from build123d import *

# Parameters (mm, degrees)
SKETCH1_W           = 85.5
SKETCH1_H           = 85.5
BOSS_EXTRUDE1_DEPTH = 3
FILLET1_R           = 2
SKETCH3_R           = 1.85
CUT_EXTRUDE1_DEPTH  = 10
SKETCH4_R           = 2.5
SKETCH4_R_2         = 1.85
CUT_EXTRUDE2_DEPTH  = 10


with BuildPart() as part:
    # Sketch1 → Boss-Extrude1 (new body)
    with BuildSketch(Plane(origin=(0, 0, 0), x_dir=(1, 0, 0), z_dir=(0, 1, 0))):
        Rectangle(SKETCH1_W, SKETCH1_H)
    extrude(amount=BOSS_EXTRUDE1_DEPTH)

    # Fillet1
    fillet1_edges = [part.edges().sort_by_distance(p)[0] for p in [
        (-42.75, 1.5, -42.75),
        (42.75, 1.5, -42.75),
        (42.75, 1.5, 42.75),
        (-42.75, 1.5, 42.75),
    ]]
    fillet(fillet1_edges, radius=FILLET1_R)

    # Sketch3 → Cut-Extrude1 (cut)
    with BuildSketch(Plane(origin=(0, 3, 0), x_dir=(1, 0, 0), z_dir=(0, 1, 0))):
        with Locations(Location((-25, 39, 0), (0, 0, 270))):
            Circle(SKETCH3_R)
        with Locations(Location((25, 39, 0), (0, 0, 270))):
            Circle(SKETCH3_R)
        with Locations(Location((25, -39, 0), (0, 0, 270))):
            Circle(SKETCH3_R)
        with Locations(Location((-25, -39, 0), (0, 0, 270))):
            Circle(SKETCH3_R)
    extrude(amount=-CUT_EXTRUDE1_DEPTH, mode=Mode.SUBTRACT)

    # Sketch4 → Cut-Extrude2 (cut)
    with BuildSketch(Plane(origin=(0, 3, 0), x_dir=(1, 0, 0), z_dir=(0, 1, 0))):
        with Locations(Location((-12.5, 10, 0), (0, 0, 270))):
            Circle(SKETCH4_R)
        with Locations(Location((-12.5, -10, 0), (0, 0, 270))):
            Circle(SKETCH4_R)
        with Locations(Location((12.5, 10, 0), (0, 0, 270))):
            Circle(SKETCH4_R)
        with Locations(Location((12.5, -10, 0), (0, 0, 270))):
            Circle(SKETCH4_R)
        with Locations(Location((-34.25, 16.7, 0), (0, 0, 270))):
            Circle(SKETCH4_R_2)
        with Locations(Location((-34.25, -10.7, 0), (0, 0, 270))):
            Circle(SKETCH4_R_2)
        with Locations(Location((34.25, -10.7, 0), (0, 0, 270))):
            Circle(SKETCH4_R_2)
        with Locations(Location((34.25, 16.7, 0), (0, 0, 270))):
            Circle(SKETCH4_R_2)
    extrude(amount=-CUT_EXTRUDE2_DEPTH, mode=Mode.SUBTRACT)


solid = part.part
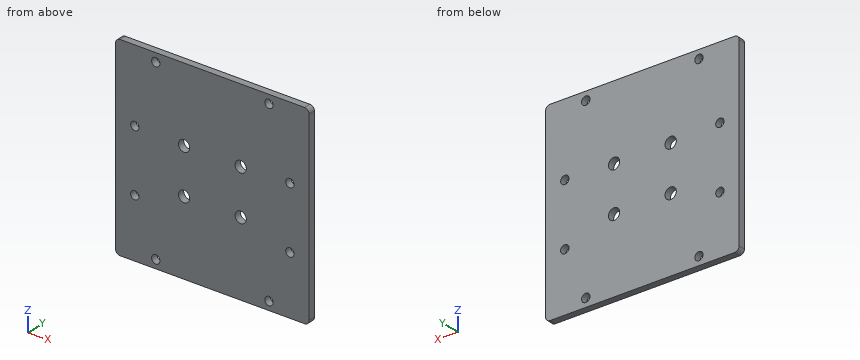
The model under review builds one solid part; all positions refer to its coordinate system, in mm. Coordinates: 2 decimals unless noted, no trailing zeros. Loops run counter-clockwise (first coordinate to the right, second up) from the corner with the lowest first, then second, coordinate; pieces in that order, holes last. Notation, with made-up numbers: M 65.25,-39 L 82.25,-39 A13 ccw 82.25,-33 Z; hole C 31.5,-39.75 d8. An arc over 180 degrees is marked long. Put each result on its own line as item: value. Start each with the question number.
Q1. Clearance check with a flat-ended pin moving along its axis: pin 1 (2 mm diameter, centred on x = 25, z = 39, fed in from +Y). State where the tip first meets the part, or that it passes through.
Q2. Add section D-D (z = 10.7). Write out the cut boundary in (x, y).
Q3. Add section B-B (z = -8.5). Write out the cut boundary in (x, y), and give its area (4 significant figures).
Q4. Add section C-C (y = 0.55). Count the separate pieces of the cut face and the enclosed holes in it, and give its area (3 significant figures).
Q5. Add section A-A (x = 12.5). Write out the cut boundary in (y, z), and give its area (4 significant figures).
Q6. Wall thickness on line 1 (Z direction, x = -13, y = 2.7); line 2 (X direction, y = 2.3, z = 10); line 3 (X direction, y = 1, z = 10.7): over which ranges is each line inside the solid? List them lowest first.
Answers:
1. pin 1: passes through
2. outline: M -42.75,0 L -36.1,0 L -36.1,3 L -42.75,3 Z; M -32.4,0 L -14.9,0 L -14.9,3 L -32.4,3 Z; M -10.1,0 L 10.1,0 L 10.1,3 L -10.1,3 Z; M 14.9,0 L 32.4,0 L 32.4,3 L 14.9,3 Z; M 36.1,0 L 42.75,0 L 42.75,3 L 36.1,3 Z
3. outline: M -42.75,0 L -14.5,0 L -14.5,3 L -42.75,3 Z; M -10.5,0 L 10.5,0 L 10.5,3 L -10.5,3 Z; M 14.5,0 L 42.75,0 L 42.75,3 L 14.5,3 Z
3. area: 232.5 mm^2
4. separate pieces: 1
4. enclosed holes: 12
4. area: 7,140 mm^2
5. outline: M 0,-42.75 L 3,-42.75 L 3,-12.5 L 0,-12.5 Z; M 0,-7.5 L 3,-7.5 L 3,7.5 L 0,7.5 Z; M 0,12.5 L 3,12.5 L 3,42.75 L 0,42.75 Z
5. area: 226.5 mm^2
6. line 1: z = -42.75 to -12.45, -7.55 to 7.55, 12.45 to 42.75
6. line 2: x = -42.75 to -35.96, -32.54 to -15, -10 to 10, 15 to 32.54, 35.96 to 42.75
6. line 3: x = -42.75 to -36.1, -32.4 to -14.9, -10.1 to 10.1, 14.9 to 32.4, 36.1 to 42.75
